Source: three-view drawing plus pictorial views. Frame: mm from the lowest corner of the part. A direction names the side the tool comes from. Give positions to 0.01 mm unless a question says otherwise; leave off trailing zeros. Order: outer loops, then holes, each group sorted by start corner. A loop starts at its lowest first (then second) coordinate and runs counter-clockwise, first axis right, second up.
1) First-contact query: P1, Ø1.5, axis at x = 50.5, y = 39, coming from the -Z side; P2, Ø8, axis at x = 40.5, y = 26, coming from the -Z side; P3, Ø6, axis at x = 71.5, y = 15.5, coming from the +Z side; P4, Ø2, axis at x = 43, z = 20.5, coming from the -Y side. Flat tips, straight axial feed; report the tip coordinate or a pass-through.
2) Material intervals for line 1 (Z direction, x = 48, y = 5.5); line 2 (Z direction, x = 48, y = 34); line 3 (Y direction, x = 67, z = 31.5), sorted ascending.
3) Section C-C, the plane y = 29. Return loops of the section in (x, z), plus the area to 3 significant figures.
4) Access query for the marked faces 4 and 5. Directions: +Z, -Z, +X, -X, +Y, -Y. A direction counts if a zero-diameter tool reaches every point of the face in a straight line with its end or side. Return the directions, or none.
5) Draft query along X for the marked faces 1, 2 and 3. Return one class per face: released by +X, released by -X, zero draft, split by the parting line, or undercut.
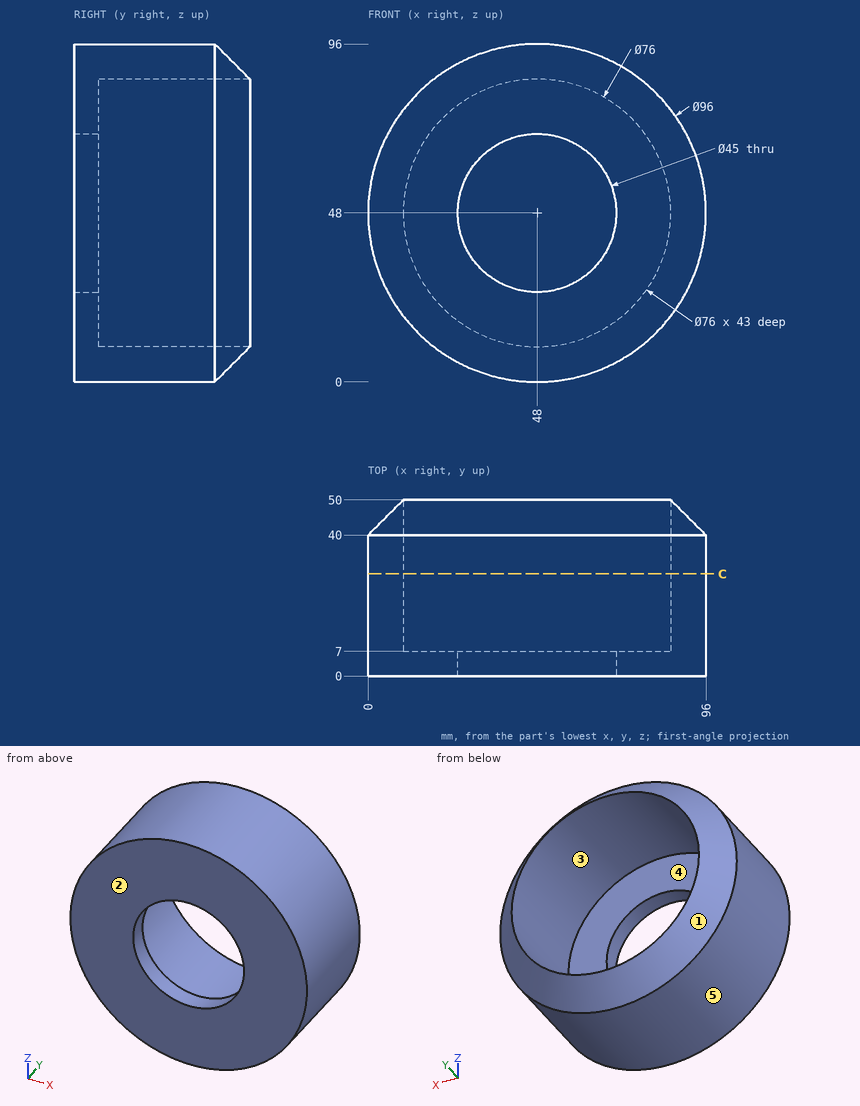
From the geometry:
1. P1: stops at z = 0.03
1. P2: stops at z = 0.13
1. P3: stops at z = 91.4
1. P4: stops at y = 0
2. line 1: z = 0 to 25.5, 70.5 to 96
2. line 2: z = 0 to 10, 86 to 96
2. line 3: y = 0 to 7
3. outline: circle Ø96 at (48, 48); hole circle Ø76 at (48, 48)
3. area: 2,700 mm2
4. face 4: +Y
4. face 5: +Y, -Y
5. face 1: split by the parting line
5. face 2: zero draft
5. face 3: undercut
